Autodesk Inventor part; units mm, degrees
ref_plane "YZ Plane" through (0, 0, 0) normal (1, 0, 0) x (0, 1, 0)
ref_plane "XZ Plane" through (0, 0, 0) normal (0, 1, 0) x (-1, 0, 0)
ref_plane "XY Plane" through (0, 0, 0) normal (0, 0, 1) x (1, 0, 0)
sketch "Sketch1" plane through (0, 0, 0) normal (0, 0, 1) x (1, 0, 0)
  line L0 (37.7292, 11.7639) -> (29.5714, 17.4761)
  line L1 (29.5714, 17.4761) -> (23.2272, 20.4344)
  line L2 (23.2272, 20.4344) -> (17.4366, 20.4344)
  line L3 (17.4366, 20.4344) -> (11.251, 17.55)
  arc A0 (11.251, 17.55) -> (10.9491, 17.3757) centre (12.0963, 15.7374) ccw
  line L4 (10.9491, 17.3757) -> (2.9346, 11.7639)
  arc A1 (2.9346, 11.7639) -> (2.0818, 10.1256) centre (4.0818, 10.1256) ccw
  line L5 (2.0818, 10.1256) -> (2.0818, 3.1667)
  arc A2 (2.0818, 3.1667) -> (4.0818, 1.1667) centre (4.0818, 3.1667) ccw
  line L6 (4.0818, 1.1667) -> (36.5821, 1.1667)
  arc A3 (36.5821, 1.1667) -> (38.5821, 3.1667) centre (36.5821, 3.1667) ccw
  line L7 (38.5821, 3.1667) -> (38.5821, 10.1256)
  arc A4 (38.5821, 10.1256) -> (37.7292, 11.7639) centre (36.5821, 10.1256) ccw
  circle A5 centre (8.3339, 6.1667) radius 1.6
  circle A6 centre (32.3301, 6.1667) radius 1.6
  circle A7 centre (20.3315, 13.1667) radius 4.25
  point P0 (0, 0)
extrude "Extrusion1" add sketch "Sketch1" along normal blind 6
thread "Thread1"
properties part number "pshfit-mount-acrylic"
Geometry: final body of the model. Coordinates: model frame, mm. Coordinates: 2 decimals unless noted, no trailing zeros. Order: outer loops, then holes, each group sorted by start corner. A loop starts at its lowest first (then second) coordinate and runs counter-clockwise, first axis right, second up. Notation, with made-up numbers: (46.25, 48) - (76.25, 48) arc R9 cw to (76.25, 61) - close; hole circle Ø6 at (22, 9). An arc over 180 degrees is marked (long way). Write each question's results on one line, items separated by ' | '.
1) Section D-D, the plane y = 18.25. Return loops of the section in (x, z), plus the area to 3 significant figures.
Results list:
outline: (12.75, 0) - (27.91, 0) - (27.91, 6) - (12.75, 6) - close | area: 91.0 mm^2
2) Pull-direction query (X, two-part tool) for faces 1 (the flat face through (26.444, 18.935, 2.958)), 2 (the cylindrical face through (33.8, 6.8, 3)), 3 (the cylindrical face through (17.199, 10.294, 2.958)), 4 (the flat face through (20, 7, 0)); classes: pulls with the +X half, pulls with the -X half, needs draft (parallel to the pull), parting line crosses it, or undercut.
Results list:
face 1: pulls with the +X half | face 2: undercut | face 3: undercut | face 4: needs draft
3) Line query: line 1 (X direction, y = 6, z = 3); line 2 (X direction, y = 5.5, z = 1.7); line 3 (Y direction, x = 11, z = 1.4). Output: solid intervals per line, ascending. Write a range as from..to.
Results list:
line 1: 2.08..6.74, 9.93..30.74, 33.92..38.58 | line 2: 2.08..6.88, 9.79..30.88, 33.78..38.58 | line 3: 1.17..17.41
4) Section C-C, the plane z = 3.4. Return loops of the section in (x, y), plus the area to 3 significant figures.
Results list:
outline: (2.08, 3.17) arc R2 ccw to (4.08, 1.17) - (36.58, 1.17) arc R2 ccw to (38.58, 3.17) - (38.58, 10.13) arc R2 ccw to (37.73, 11.76) - (29.57, 17.48) - (23.23, 20.43) - (17.44, 20.43) - (11.25, 17.55) arc R2 ccw to (10.95, 17.38) - (2.93, 11.76) arc R2 ccw to (2.08, 10.13) - close; hole circle Ø3.2 at (8.33, 6.17); hole circle Ø8.5 at (20.33, 13.17); hole circle Ø3.2 at (32.33, 6.17) | area: 499 mm^2
5) Pin query (flat end, axial travel): pin 1 (3 mm diameter, centred on x = 15.5, y = 5.5, fed in from -Z). Return the tip coordinate at first contact, or that it passes through.
Results list:
pin 1: z = 0
6) Section A-A, the plane x = 7.5. Return loops of the section in (y, z), plus the area to 3 significant figures.
Results list:
outline: (1.17, 0) - (4.8, 0) - (4.8, 6) - (1.17, 6) - close; (7.53, 0) - (14.96, 0) - (14.96, 6) - (7.53, 6) - close | area: 66.4 mm^2
7) Section B-B, the plane y = 15.25. Return loops of the section in (x, z).
Results list:
outline: (7.91, 0) - (16.63, 0) - (16.63, 6) - (7.91, 6) - close; (24.04, 0) - (32.75, 0) - (32.75, 6) - (24.04, 6) - close
